Part print with two shaded views. Sizes in mm from the minimum x, y, z corner. Give positions to 0.01 mm unless a question says otherwise; leave off trailing zeros. Write each loop counter-clockwise with the first axis right and the second up, starting at its lowest first coordinate (ties: lowest second). Pieces come first, ordered by that corner, then holes. Notation, with made-up numbers: (-20.75, 21.5) - (22.25, 21.5) arc R34 cw to (22.25, 56.5) - close; hole circle Ø4 at (86, -34.5). An arc over 180 degrees is marked (long way). Answer as a JSON object with one key per item and string values.
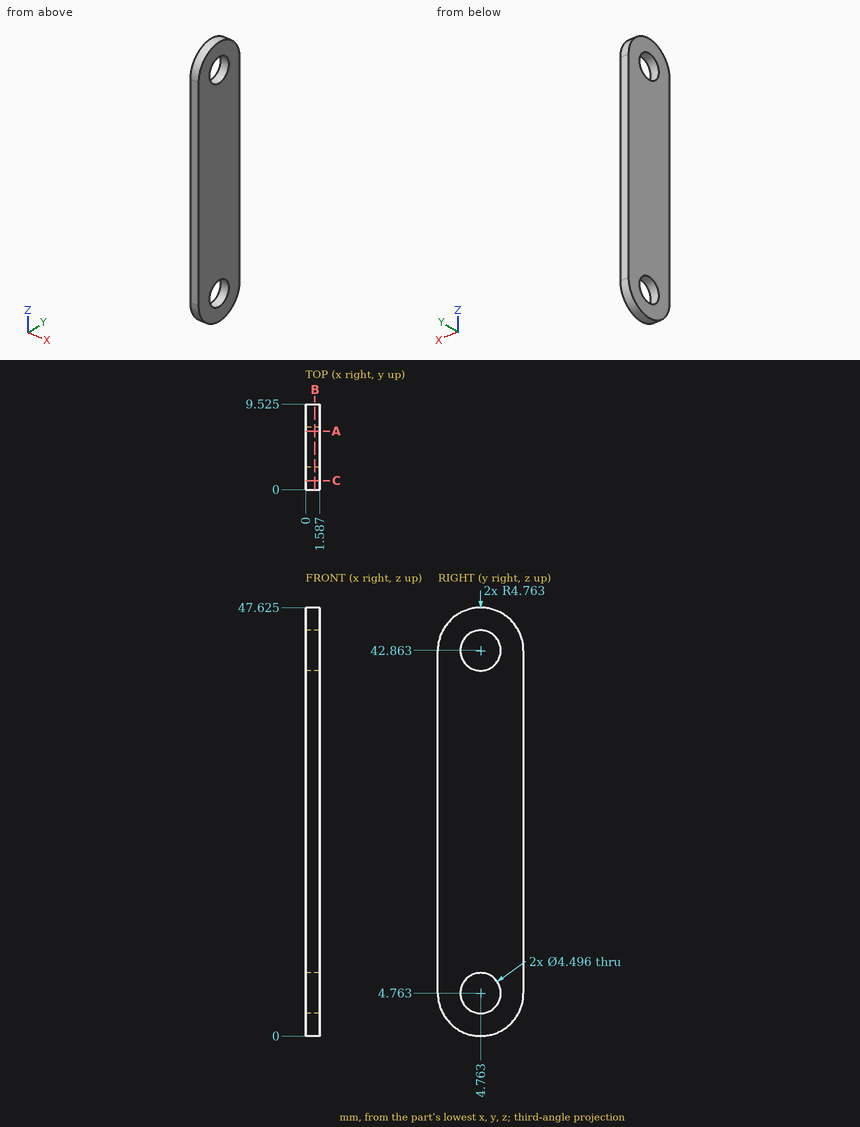
(1) Saw through at C-C, the plane y = 1. Give the cut face in (x, z).
Answer key:
{"outline": "(0, 1.84) - (1.59, 1.84) - (1.59, 45.78) - (0, 45.78) - close"}
(2) Saw through at B-B, the plane x = 1.05. Give the cut face in (y, z) (1 decimal).
Answer key:
{"outline": "(0, 4.8) arc R4.8 ccw to (9.5, 4.8) - (9.5, 42.9) arc R4.8 ccw to (0, 42.9) - close; hole circle Ø4.5 at (4.8, 4.8); hole circle Ø4.5 at (4.8, 42.9)"}
(3) Saw through at A-A, the plane y = 6.5. Give the cut face in (x, z).
Answer key:
{"outline": "(0, 0.33) - (1.59, 0.33) - (1.59, 3.34) - (0, 3.34) - close; (0, 6.19) - (1.59, 6.19) - (1.59, 41.44) - (0, 41.44) - close; (0, 44.29) - (1.59, 44.29) - (1.59, 47.3) - (0, 47.3) - close"}
(4) Probe L1, parallel to Z at x = 1.4, y = 6 (1 decimal); L2, parallel to Z at x = 1.05, y = 5.5 (1 decimal); L3, parallel to Y at x = 1.1, z = 44 (1 decimal). List the from-to ranges inside material, lowest first. Write a range as [from, to].
Answer key:
{"L1": "z = [0.2, 2.9], [6.6, 41], [44.7, 47.5]", "L2": "z = [0.1, 2.6], [6.9, 40.7], [45, 47.6]", "L3": "y = [0.1, 2.8], [6.7, 9.4]"}
